Geometry check sheet. Reference: the model listing, model coordinates, mm. A direction names the side the tool comes from. Coordinates: 2 decimals unless noted, no trailing zeros. Order: outer loops, then holes, each group sorted by start corner. A loop starts at its lowest first (then second) coordinate and runs counter-clockwise, first axis right, second up. Notation, with made-up numbers: (37, 65) - (87, 65) arc R31 ccw to (87, 91) - close; hole circle Ø7 at (-38.75, 9). An arc over 180 degrees is marked (long way). Return JSON: item names as keys, results as strings. Group by question number.
Item 1: Section check A-A on y = 2. Give the number of separate pieces and of enclosed holes in the cut face, then the cut area to 3 significant figures.
Item 2: Section check B-B on x = -39. Enter the section's corners in (y, z).
Item 3: Draft check along Z on faces 5 (the cylindrical face through (-32.69, 7.4, 33.23)), 6 (the flat face through (-34, 10, 24.09)), 7 (the cylindrical face through (-32.69, 7.4, -33.23)). Enter one of: pulls with the +Z half, pulls with the -Z half, needs draft (parallel to the pull), parting line crosses it, or undercut.
Item 4: Section check D-D on z = 14.5. Enter the section's corners in (x, y), then the cut area to 3 significant figures.
Item 5: Gauge pin test, flat ends, axial feed: pin 1 (5.5 mm diameter, centred on y = 9, z = 22.5, fed in from +X); pin 2 (6 mm diameter, centred on x = -21, z = -16, fed in from +Y); pin 3 (1.6 mm diameter, centred on x = -43, y = 7, fed in from -Z). Record the tip position at first contact, or that the pin passes through.
Item 6: Tool access check on faces 1 (the flat face through (-39, 10, -19.09)), 2 (the flat face through (-43, 8, 19.09)), 3 (the flat face through (-42.34, 7, 22)), 4 (the flat face through (-27, 4, 28.54)). Record the directions out of +Z, -Z, +X, -X, +Y, -Y that give a thin tool (end or side, any length) a straight path to the whole face; none if there is none.
Item 7: Scan lines: probe 1 along X at (y, z) = (6.25, 29.09); probe 2 along Z at (x, y) = (-41.5, 6); probe 3 along Y at (x, z) = (-16.5, -13.5). Record each from-to range of solid material in increasing order.
from build123d import *

# Parameters (mm, degrees)
SKETCH2_W          = 93.58
SKETCH2_H          = 68.18
BASE_DEPTH         = 5
SKETCH2_7_W        = 4.45
SKETCH2_7_H        = 4.45
SKETCH2_7_H_2      = 5
SKETCH2_7_W_2      = 5
SKETCH2_7_H_3      = 1.1
SKETCH2_7_W_3      = 1.1
WALLS_DEPTH        = 15
SKETCH2_10_W       = 1.1
SKETCH2_10_H       = 5
SKETCH2_10_H_2     = 38.18
SKETCH2_10_W_2     = 5
SKETCH2_10_H_3     = 1.1
SKETCH2_10_W_3     = 63.58
ACRYLIC_CUT_DEPTH  = 60.803279174
SKETCH4_W          = 63.58
SKETCH4_H          = 4.45
SKETCH4_W_2        = 4.45
SKETCH4_H_2        = 38.18
CUT_EXTRUDE2_DEPTH = 5
SKETCH5_R          = 2.25
SCREW_HOLES_DEPTH  = 5
FILLET1_R          = 5
FILLET2_R          = 3
SKETCH8_R          = 2
CUT_EXTRUDE3_DEPTH = 15
SKETCH7_W          = 13.03
SKETCH7_H          = 57.08
SKETCH7_W_2        = 40
SKETCH7_H_2        = 68.18
TOP_CUT_DEPTH      = 60.803279174
FILLET4_R          = 5


with BuildPart() as part:
    # Sketch2 → Base (new body)
    with BuildSketch(Plane(origin=(0, 0, 0), x_dir=(1, 0, 0), z_dir=(0, 1, 0))):
        Rectangle(SKETCH2_W, SKETCH2_H)
    extrude(amount=BASE_DEPTH)

    # Sketch2<7> → Walls (add)
    with BuildSketch(Plane(origin=(0, 0, 0), x_dir=(1, 0, 0), z_dir=(0, 1, 0))):
        with Locations((-39.015, 26.315)):
            Rectangle(SKETCH2_7_W, SKETCH2_7_H)
        with Locations((-39.015, 21.59)):
            Rectangle(SKETCH2_7_W, SKETCH2_7_H_2)
        with Locations((-44.565, 21.59)):
            Rectangle(SKETCH2_7_W, SKETCH2_7_H_2)
        with Locations((-44.565, 26.315)):
            Rectangle(SKETCH2_7_W, SKETCH2_7_H)
        with Locations((-44.565, 31.865)):
            Rectangle(SKETCH2_7_W, SKETCH2_7_H)
        with Locations((-39.015, 31.865)):
            Rectangle(SKETCH2_7_W, SKETCH2_7_H)
        with Locations((-34.29, 31.865)):
            Rectangle(SKETCH2_7_W_2, SKETCH2_7_H)
        with Locations((-34.29, 26.315)):
            Rectangle(SKETCH2_7_W_2, SKETCH2_7_H)
        with Locations((-34.29, 29.09)):
            Rectangle(SKETCH2_7_W_2, SKETCH2_7_H_3)
        with Locations((-39.015, 29.09)):
            Rectangle(SKETCH2_7_W, SKETCH2_7_H_3)
        with Locations((-44.565, 29.09)):
            Rectangle(SKETCH2_7_W, SKETCH2_7_H_3)
        with Locations((-41.79, 31.865)):
            Rectangle(SKETCH2_7_W_3, SKETCH2_7_H)
        with Locations((-41.79, 26.315)):
            Rectangle(SKETCH2_7_W_3, SKETCH2_7_H)
        with Locations((-41.79, 29.09)):
            Rectangle(SKETCH2_7_W_3, SKETCH2_7_H_3)
        with Locations((-41.79, 21.59)):
            Rectangle(SKETCH2_7_W_3, SKETCH2_7_H_2)
        with Locations((-34.29, -26.315)):
            Rectangle(SKETCH2_7_W_2, SKETCH2_7_H)
        with Locations((-34.29, -31.865)):
            Rectangle(SKETCH2_7_W_2, SKETCH2_7_H)
        with Locations((-39.015, -31.865)):
            Rectangle(SKETCH2_7_W, SKETCH2_7_H)
        with Locations((-39.015, -26.315)):
            Rectangle(SKETCH2_7_W, SKETCH2_7_H)
        with Locations((-44.565, -26.315)):
            Rectangle(SKETCH2_7_W, SKETCH2_7_H)
        with Locations((-44.565, -31.865)):
            Rectangle(SKETCH2_7_W, SKETCH2_7_H)
        with Locations((-44.565, -29.09)):
            Rectangle(SKETCH2_7_W, SKETCH2_7_H_3)
        with Locations((-41.79, -31.865)):
            Rectangle(SKETCH2_7_W_3, SKETCH2_7_H)
        with Locations((-41.79, -29.09)):
            Rectangle(SKETCH2_7_W_3, SKETCH2_7_H_3)
        with Locations((-41.79, -26.315)):
            Rectangle(SKETCH2_7_W_3, SKETCH2_7_H)
        with Locations((-44.565, -21.59)):
            Rectangle(SKETCH2_7_W, SKETCH2_7_H_2)
        with Locations((-39.015, -21.59)):
            Rectangle(SKETCH2_7_W, SKETCH2_7_H_2)
        with Locations((-41.79, -21.59)):
            Rectangle(SKETCH2_7_W_3, SKETCH2_7_H_2)
        with Locations((-39.015, -29.09)):
            Rectangle(SKETCH2_7_W, SKETCH2_7_H_3)
        with Locations((-34.29, -29.09)):
            Rectangle(SKETCH2_7_W_2, SKETCH2_7_H_3)
        with Locations((39.015, -21.59)):
            Rectangle(SKETCH2_7_W, SKETCH2_7_H_2)
        with Locations((44.565, -21.59)):
            Rectangle(SKETCH2_7_W, SKETCH2_7_H_2)
        with Locations((44.565, -26.315)):
            Rectangle(SKETCH2_7_W, SKETCH2_7_H)
        with Locations((39.015, -26.315)):
            Rectangle(SKETCH2_7_W, SKETCH2_7_H)
        with Locations((34.29, -31.865)):
            Rectangle(SKETCH2_7_W_2, SKETCH2_7_H)
        with Locations((39.015, -31.865)):
            Rectangle(SKETCH2_7_W, SKETCH2_7_H)
        with Locations((44.565, -31.865)):
            Rectangle(SKETCH2_7_W, SKETCH2_7_H)
        with Locations((41.79, -31.865)):
            Rectangle(SKETCH2_7_W_3, SKETCH2_7_H)
        with Locations((44.565, -29.09)):
            Rectangle(SKETCH2_7_W, SKETCH2_7_H_3)
        with Locations((41.79, -26.315)):
            Rectangle(SKETCH2_7_W_3, SKETCH2_7_H)
        with Locations((41.79, -21.59)):
            Rectangle(SKETCH2_7_W_3, SKETCH2_7_H_2)
        with Locations((34.29, -26.315)):
            Rectangle(SKETCH2_7_W_2, SKETCH2_7_H)
        with Locations((34.29, -29.09)):
            Rectangle(SKETCH2_7_W_2, SKETCH2_7_H_3)
        with Locations((39.015, -29.09)):
            Rectangle(SKETCH2_7_W, SKETCH2_7_H_3)
        with Locations((41.79, -29.09)):
            Rectangle(SKETCH2_7_W_3, SKETCH2_7_H_3)
        with Locations((34.29, 26.315)):
            Rectangle(SKETCH2_7_W_2, SKETCH2_7_H)
        with Locations((34.29, 31.865)):
            Rectangle(SKETCH2_7_W_2, SKETCH2_7_H)
        with Locations((39.015, 31.865)):
            Rectangle(SKETCH2_7_W, SKETCH2_7_H)
        with Locations((39.015, 26.315)):
            Rectangle(SKETCH2_7_W, SKETCH2_7_H)
        with Locations((44.565, 26.315)):
            Rectangle(SKETCH2_7_W, SKETCH2_7_H)
        with Locations((44.565, 31.865)):
            Rectangle(SKETCH2_7_W, SKETCH2_7_H)
        with Locations((44.565, 21.59)):
            Rectangle(SKETCH2_7_W, SKETCH2_7_H_2)
        with Locations((39.015, 21.59)):
            Rectangle(SKETCH2_7_W, SKETCH2_7_H_2)
        with Locations((41.79, 21.59)):
            Rectangle(SKETCH2_7_W_3, SKETCH2_7_H_2)
        with Locations((41.79, 26.315)):
            Rectangle(SKETCH2_7_W_3, SKETCH2_7_H)
        with Locations((41.79, 31.865)):
            Rectangle(SKETCH2_7_W_3, SKETCH2_7_H)
        with Locations((44.565, 29.09)):
            Rectangle(SKETCH2_7_W, SKETCH2_7_H_3)
        with Locations((41.79, 29.09)):
            Rectangle(SKETCH2_7_W_3, SKETCH2_7_H_3)
        with Locations((39.015, 29.09)):
            Rectangle(SKETCH2_7_W, SKETCH2_7_H_3)
        with Locations((34.29, 29.09)):
            Rectangle(SKETCH2_7_W_2, SKETCH2_7_H_3)
    extrude(amount=WALLS_DEPTH)

    # Sketch2<10> → Acrylic Cut (cut, through all)
    with BuildSketch(Plane(origin=(0, 0, 0), x_dir=(1, 0, 0), z_dir=(0, 1, 0))):
        with Locations((41.79, -21.59)):
            Rectangle(SKETCH2_10_W, SKETCH2_10_H)
        with Locations((41.79, 0)):
            Rectangle(SKETCH2_10_W, SKETCH2_10_H_2)
        with Locations((34.29, -29.09)):
            Rectangle(SKETCH2_10_W_2, SKETCH2_10_H_3)
        with Locations((0, -29.09)):
            Rectangle(SKETCH2_10_W_3, SKETCH2_10_H_3)
        with Locations((41.79, 21.59)):
            Rectangle(SKETCH2_10_W, SKETCH2_10_H)
        with Locations((34.29, 29.09)):
            Rectangle(SKETCH2_10_W_2, SKETCH2_10_H_3)
        with Locations((0, 29.09)):
            Rectangle(SKETCH2_10_W_3, SKETCH2_10_H_3)
        with Locations((-34.29, 29.09)):
            Rectangle(SKETCH2_10_W_2, SKETCH2_10_H_3)
        with Locations((-41.79, 21.59)):
            Rectangle(SKETCH2_10_W, SKETCH2_10_H)
        with Locations((-41.79, 0)):
            Rectangle(SKETCH2_10_W, SKETCH2_10_H_2)
        with Locations((-41.79, -21.59)):
            Rectangle(SKETCH2_10_W, SKETCH2_10_H)
        with Locations((-34.29, -29.09)):
            Rectangle(SKETCH2_10_W_2, SKETCH2_10_H_3)
    extrude(amount=ACRYLIC_CUT_DEPTH, mode=Mode.SUBTRACT)

    # Sketch4 → Cut-Extrude2 (cut)
    with BuildSketch(Plane(origin=(0, 5, 0), x_dir=(1, 0, 0), z_dir=(0, 1, 0))):
        with Locations((0, -31.865)):
            Rectangle(SKETCH4_W, SKETCH4_H)
        with Locations((44.565, 0)):
            Rectangle(SKETCH4_W_2, SKETCH4_H_2)
        with Locations((0, 31.865)):
            Rectangle(SKETCH4_W, SKETCH4_H)
        with Locations((-44.565, 0)):
            Rectangle(SKETCH4_W_2, SKETCH4_H_2)
    extrude(amount=-CUT_EXTRUDE2_DEPTH, mode=Mode.SUBTRACT)

    # Sketch5 → Screw Holes (add)
    with BuildSketch(Plane(origin=(0, 5, 0), x_dir=(1, 0, 0), z_dir=(0, 1, 0))):
        with Locations(Location((36.79, -10.16, 0), (0, 0, 90))):
            Circle(SKETCH5_R)
        with Locations(Location((16.79, -10.16, 0), (0, 0, 90))):
            Circle(SKETCH5_R)
        with Locations(Location((26.79, 19.64, 0), (0, 0, 90))):
            Circle(SKETCH5_R)
    extrude(amount=SCREW_HOLES_DEPTH)

    # Fillet1
    fillet1_edges = [part.edges().sort_by_distance(p)[0] for p in [
        (-46.79, 7.5, 34.09),
        (46.79, 7.5, 34.09),
        (46.79, 7.5, -34.09),
        (-46.79, 7.5, -34.09),
    ]]
    fillet(fillet1_edges, radius=FILLET1_R)

    # Fillet2
    fillet2_edges = [part.edges().sort_by_distance(p)[0] for p in [
        (31.79, 7.5, -34.09),
        (46.79, 7.5, -19.09),
        (-46.79, 7.5, -19.09),
        (-31.79, 7.5, -34.09),
        (-46.79, 7.5, 19.09),
        (-31.79, 7.5, 34.09),
        (31.79, 7.5, 34.09),
        (46.79, 7.5, 19.09),
    ]]
    fillet(fillet2_edges, radius=FILLET2_R)

    # Sketch8 → Cut-Extrude3 (cut)
    with BuildSketch(Plane(origin=(0, 15, 0), x_dir=(1, 0, 0), z_dir=(0, 1, 0))):
        with Locations(Location((41.79, -29.09, 0), (0, 0, 270))):
            Circle(SKETCH8_R)
        with Locations(Location((-41.79, -29.09, 0), (0, 0, 90))):
            Circle(SKETCH8_R)
        with Locations(Location((-41.79, 29.09, 0), (0, 0, 270))):
            Circle(SKETCH8_R)
        with Locations(Location((41.79, 29.09, 0), (0, 0, 90))):
            Circle(SKETCH8_R)
    extrude(amount=-CUT_EXTRUDE3_DEPTH, mode=Mode.SUBTRACT)

    # Sketch7 → Top Cut (cut, through all)
    with BuildSketch(Plane.XZ):
        with Locations((0.275, 0)):
            Rectangle(SKETCH7_W, SKETCH7_H)
        with Locations((26.79, 0)):
            Rectangle(SKETCH7_W_2, SKETCH7_H_2)
    extrude(amount=-TOP_CUT_DEPTH, mode=Mode.SUBTRACT)

    # Fillet4
    fillet4_edges = [part.edges().sort_by_distance(p)[0] for p in [
        (-6.24, 2.5, 28.54),
        (-6.24, 2.5, -28.54),
    ]]
    fillet(fillet4_edges, radius=FILLET4_R)


solid = part.part
Computed:
{
 "1": {"separate pieces": "1", "enclosed holes": "2", "area": "2,190 mm²"},
 "2": {"outline": "(0, -34.09) - (15, -34.09) - (15, -19.09) - (5, -19.09) - (5, 19.09) - (15, 19.09) - (15, 34.09) - (0, 34.09) - close"},
 "3": {"face 5": "pulls with the +Z half", "face 6": "undercut", "face 7": "pulls with the -Z half"},
 "4": {"outline": "(-41.24, 0) - (-6.24, 0) - (-6.24, 5) - (-41.24, 5) - close", "area": "175 mm²"},
 "5": {"pin 1": "stops at x = -31.79", "pin 2": "stops at y = 5", "pin 3": "stops at z = -34.07"},
 "6": {"face 1": "+X, -X, +Y", "face 2": "-X, +Y, -Y", "face 3": "+Y, -Y", "face 4": "+X, +Y, -Y"},
 "7": {"probe 1": "x = -46.79 to -43.79, -39.79 to -36.79", "probe 2": "z = -34.09 to -31.07, -27.11 to -24.09, 24.09 to 27.11, 31.07 to 34.09", "probe 3": "y = 0 to 5"}
}
